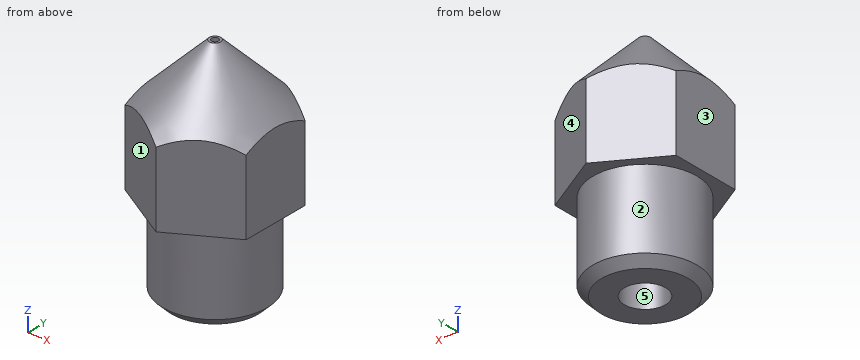
from build123d import *

# Parameters (mm, degrees)
SKETCH2_R          = 8.325
CUT_EXTRUDE2_DEPTH = 10
CHAMFER1_SIZE      = 0.5


with BuildPart() as part:
    # Sketch1 → Revolve1 (revolve)
    with BuildSketch(Plane(origin=(0, 0, 0), x_dir=(1, 0, 0), z_dir=(0, 1, 0)), mode=Mode.PRIVATE) as revolve1_sk:
        Polygon((1.19, 0), (3, 0), (3, -5), (8.325, -5), (0.325, -13), (0.2, -13), (0.2, -12.5), (1.19, -10.785269701), align=None)
    revolve(revolve1_sk.sketch.rotate(Axis((0, 0, 0), (0, 0, 1)), 180), axis=Axis((0, 0, 0), (0, 0, 1)))

    # Sketch2 → Cut-Extrude2 (cut)
    with BuildSketch(Plane(origin=(0, 0, 5), x_dir=(-1, 0, 0), z_dir=(0, 0, -1))):
        Circle(SKETCH2_R)
        Polygon((3.5, 2.020725942), (0, 4.041451884), (-3.5, 2.020725942), (-3.5, -2.020725942), (0, -4.041451884), (3.5, -2.020725942), align=None, mode=Mode.SUBTRACT)
    extrude(amount=-CUT_EXTRUDE2_DEPTH, mode=Mode.SUBTRACT)

    # Chamfer1
    chamfer1_edges = [part.edges().sort_by_distance(p)[0] for p in [
        (3, 0, 0),
    ]]
    chamfer(chamfer1_edges, length=CHAMFER1_SIZE)


solid = part.part
Can you work these out from the model? Positions are in its coordinate system, mm. Face numbers are marked on the shaded views. A direction names the side the tool comes from. Give positions to 0.01 mm unless a question says otherwise; leave off trailing zeros. Order: outer loops, then holes, each group sorted by start corner. A loop starts at its lowest first (then second) coordinate and runs counter-clockwise, first axis right, second up. Notation, with made-up numbers: M 53.25,-16 L 85.25,-16 A19 ccw 85.25,-11 Z; hole C -15.75,78.25 d6. An arc over 180 degrees is marked long. One line per item, written item: value.
Item 1: If we section it at B-B on z = 6.75: Write out the boundary of the cut face in (x, y).
Verdict:
outline: M -3.5,-2.02 L 0,-4.04 L 3.5,-2.02 L 3.5,2.02 L 0,4.04 L -3.5,2.02 Z; hole C 0,0 d2.38
Item 2: If we mould it in two halves opening along X, with no side actions, what happens to the marked faces 3, 4 and 5? For each: pulls with the +X half, pulls with the -X half, needs draft (parallel to the pull), parting line crosses it, or undercut.
Verdict:
face 3: pulls with the -X half
face 4: pulls with the +X half
face 5: undercut
Item 3: For pin 1 (2 mm diameter, centred on x = -2, y = 3, fed in from -Z); pin 2 (3 mm diameter, centred on x = -2.5, y = -2.5, fed in from +Z); pin 3 (1.9 mm diameter, centred on x = 0, y = 0, fed in from -Z), each with a flat end and sliding along its axis, tell me the tip position at first contact or that it passes through.
Verdict:
pin 1: z = 0.11
pin 2: z = 11.29
pin 3: z = 11.2
Item 4: Please list where these lines run through material, in increasing order: line 1 (Y direction, x = 0, z = 12.65) (3 decimals); line 2 (Y direction, x = 0.75, z = 9.25); line 3 (X direction, y = 0.25, z = 3.5).
Verdict:
line 1: -0.675 to -0.2, 0.2 to 0.675
line 2: -3.61 to -0.92, 0.92 to 3.61
line 3: -2.99 to -1.16, 1.16 to 2.99
Item 5: For the marked faces 1 and 2, which set-ups out of +Z, -Z, +X, -X, +Y, -Y let a thin tool reach every point of the face, with its end or its side?
Verdict:
face 1: +Z, -Z, -X, -Y
face 2: -Z
Item 6: If we section it at D-D on z = 10.5: Write out the boundary of the cut face in (x, y) (3 decimals).
Verdict:
outline: C 0,0 d5.65; hole C 0,0 d2.38
Item 7: If we section it at C-C on z = 4.75: Write out the boundary of the cut face in (x, y).
Verdict:
outline: C 0,0 d6; hole C 0,0 d2.38
Item 8: If we section it at A-A on y = 0: Write out the boundary of the cut face in (x, z) (3 decimals).
Verdict:
outline: M -3.5,5 L -3,5 L -3,0.5 L -2.5,0 L -1.19,0 L -1.19,10.785 L -0.2,12.5 L -0.2,13 L -0.325,13 L -3.5,9.825 Z; M 0.2,12.5 L 1.19,10.785 L 1.19,0 L 2.5,0 L 3,0.5 L 3,5 L 3.5,5 L 3.5,9.825 L 0.325,13 L 0.2,13 Z
